Design review of the part built by this model. Coordinates are the model's own, in mm. Round coordinates to 2 decimals unless told otherwise and drop trailing zeros. Write each loop counter-clockwise with the first axis right and the second up, starting at its lowest first coordinate (ties: lowest second). Pieces come first, ordered by that corner, then holes. Notation, with made-up numbers: (22, -27) -> (39, -27) arc R19 ccw to (39, -2) -> close; hole circle Ø11 at (69.25, 80.25). An arc over 180 degrees is marked (long way). Write item = value, one per line. Start each with the question number.
Item 1: Add section B-B, the plane z = -600. State the section outline as (x, y) points, then the cut area to 3 significant figures.
Item 2: For pin 1 Ø1.9 at (y, z) = (3.5, -443.5) entering from -X; pin 2 Ø3 at (x, y) = (1036, 3.5) entering from -Z; pin 3 Ø11.5 at (x, z) = (22.225, -92.075) entering from -Y, all flat-tipped, find the tip position at first contact; note any pin that passes through.
Item 3: Add section C-C, the plane y = 3.5. State how many separate pieces and enclosed holes the cut face has, then the cut area to 3 significant figures.
Item 4: Add section D-D, the plane x = 881.5. State the section outline as (y, z) points (3 decimals).
Item 5: To check wall thickness, follow L1, parallel to X at y = 3.25, z = -309.5; L2, parallel to X at y = 0.75, z = -594.5; L3, parallel to X at y = 1, z = -278.5. State the ranges of each line that lie inside material, in increasing order.
Item 6: Add section A-A, the plane x = 88.9. State the section outline as (y, z) points (3 decimals).
from build123d import *

# Parameters (mm, degrees)
SKETCH1_R                                     = 3.3734375
BOSS_EXTRUDE1_DEPTH                           = 6.35
SKETCH3_R                                     = 2.45745
SKETCH3_R_2                                   = 22.225
CUT_EXTRUDE2_DEPTH                            = 1264.111411604
CUT_EXTRUDE1_DEPTH                            = 1264.111411604
CSK_FOR_1_4_FLAT_HEAD_MACHINE_SCREW1_AT_COUNT = 2
CSK_FOR_1_4_FLAT_HEAD_MACHINE_SCREW1_AT_PITCH = 1022.35
CSK_FOR_1_4_FLAT_HEAD_MACHINE_SCREW1_2_COUNT  = 2
CSK_FOR_1_4_FLAT_HEAD_MACHINE_SCREW1_2_PITCH  = 203.2
CSK_FOR_1_4_FLAT_HEAD_MACHINE_SCREW1_3_COUNT  = 2
CSK_FOR_1_4_FLAT_HEAD_MACHINE_SCREW1_3_PITCH  = 1042.348196382
FILLET1_R                                     = 6.35
FILLET3_R                                     = 3.175


with BuildPart() as part:
    # Sketch1 → Boss-Extrude1 (new body)
    with BuildSketch(Plane(origin=(0, 0, 0), x_dir=(1, 0, 0), z_dir=(0, 1, 0))):
        Polygon((1016, 406.4), (1066.8, 406.4), (1066.8, 0), (0, 0), (0, 406.4), (50.8, 406.4), (50.8, 530.225), (234.95, 530.225), (234.95, 676.275), (831.85, 676.275), (831.85, 530.225), (1016, 530.225), align=None)
        with Locations(Location((22.225, 92.075, 0), (0, 0, 270))):
            Circle(SKETCH1_R, mode=Mode.SUBTRACT)
        with Locations(Location((1044.575, 92.075, 0), (0, 0, 270))):
            Circle(SKETCH1_R, mode=Mode.SUBTRACT)
        with Locations(Location((22.225, 295.275, 0), (0, 0, 270))):
            Circle(SKETCH1_R, mode=Mode.SUBTRACT)
        with Locations(Location((1044.575, 295.275, 0), (0, 0, 270))):
            Circle(SKETCH1_R, mode=Mode.SUBTRACT)
    extrude(amount=BOSS_EXTRUDE1_DEPTH)

    # Sketch3 → Cut-Extrude2 (cut, through all)
    with BuildSketch(Plane(origin=(0, 6.35, 0), x_dir=(1, 0, 0), z_dir=(0, 1, 0))):
        with Locations(Location((134.9375, 487.748914195, 0), (0, 0, 270))):
            Circle(SKETCH3_R)
        with Locations(Location((219.486424299, 515.220524995, 0), (0, 0, 270))):
            Circle(SKETCH3_R)
        with Locations(Location((59.31154, 45.87748, 0), (0, 0, 270))):
            Circle(SKETCH3_R)
        with Locations(Location((296.845703608, 123.057008284, 0), (0, 0, 270))):
            Circle(SKETCH3_R)
        with Locations(Location((534.379867216, 200.236536569, 0), (0, 0, 270))):
            Circle(SKETCH3_R)
        with Locations(Location((771.914030824, 277.416064853, 0), (0, 0, 270))):
            Circle(SKETCH3_R)
        with Locations(Location((854.075, 309.0545, 0), (0, 0, 270))):
            Circle(SKETCH3_R)
        with Locations(Location((854.075, 486.8545, 0), (0, 0, 270))):
            Circle(SKETCH3_R)
        with Locations(Location((88.9, 492.125, 0), (0, 0, 270))):
            Circle(SKETCH3_R_2)
    extrude(amount=-CUT_EXTRUDE2_DEPTH, mode=Mode.SUBTRACT)

    # Sketch2 → Cut-Extrude1 (cut, through all)
    with BuildSketch(Plane(origin=(0, 6.35, 0), x_dir=(1, 0, 0), z_dir=(0, 1, 0))):
        Polygon((310.578822168, 0), (149.225, 0), (149.225, 95.25), (171.033618902, 121.240499926), (157.061866823, 164.241131286), (247.65, 193.675), align=None)
    extrude(amount=-CUT_EXTRUDE1_DEPTH, mode=Mode.SUBTRACT)

    # Sketch5 → CSK for 1/4 Flat Head Machine Screw1 (revolve, cut)
    with BuildSketch(Plane(origin=(22.225, 0, -92.075), x_dir=(0, 0, -1), z_dir=(1, 0, 0))):
        Polygon((0, 0), (0, 6.35), (3.3782, 6.35), (3.3782, 4.536932584), (6.4389, 1.016), (6.4389, 0), align=None)
    csk_for_1_4_flat_head_machine_screw1 = revolve(axis=Axis((22.225, -6.35, -92.075), (0, 1, 0)), mode=Mode.SUBTRACT)

    # CSK for 1/4 Flat Head Machine Screw1 at: CSK for 1/4 Flat Head Machine Screw1 ×2
    with Locations(*[(i * CSK_FOR_1_4_FLAT_HEAD_MACHINE_SCREW1_AT_PITCH, 0, 0) for i in range(1, CSK_FOR_1_4_FLAT_HEAD_MACHINE_SCREW1_AT_COUNT)]):
        add(csk_for_1_4_flat_head_machine_screw1, mode=Mode.SUBTRACT)

    # CSK for 1_4 Flat Head Machine Screw1 2: CSK for 1/4 Flat Head Machine Screw1 ×2
    with Locations(*[(0, 0, -i * CSK_FOR_1_4_FLAT_HEAD_MACHINE_SCREW1_2_PITCH) for i in range(1, CSK_FOR_1_4_FLAT_HEAD_MACHINE_SCREW1_2_COUNT)]):
        add(csk_for_1_4_flat_head_machine_screw1, mode=Mode.SUBTRACT)

    # CSK for 1_4 Flat Head Machine Screw1 3: CSK for 1/4 Flat Head Machine Screw1 ×2
    with Locations(*[Vector(0.9808142840837317, 0, -0.19494445397937524) * (i * CSK_FOR_1_4_FLAT_HEAD_MACHINE_SCREW1_3_PITCH) for i in range(1, CSK_FOR_1_4_FLAT_HEAD_MACHINE_SCREW1_3_COUNT)]):
        add(csk_for_1_4_flat_head_machine_screw1, mode=Mode.SUBTRACT)

    # Fillet1
    fillet1_edges = [part.edges().sort_by_distance(p)[0] for p in [
        (0, 3.175, -406.4),
        (50.8, 3.175, -406.4),
        (50.8, 3.175, -530.225),
        (234.95, 3.175, -530.225),
        (234.95, 3.175, -676.275),
        (831.85, 3.175, -676.275),
        (831.85, 3.175, -530.225),
        (1016, 3.175, -530.225),
        (1016, 3.175, -406.4),
        (1066.8, 3.175, -406.4),
        (1066.8, 3.175, 0),
        (0, 3.175, 0),
    ]]
    fillet(fillet1_edges, radius=FILLET1_R)

    # Fillet3
    fillet3_edges = [part.edges().sort_by_distance(p)[0] for p in [
        (247.65, 3.175, -193.675),
        (310.578822168, 3.175, 0),
        (149.225, 3.175, 0),
        (149.225, 3.175, -95.25),
        (171.033618902, 3.175, -121.240499926),
        (157.061866823, 3.175, -164.241131286),
    ]]
    fillet(fillet3_edges, radius=FILLET3_R)


solid = part.part
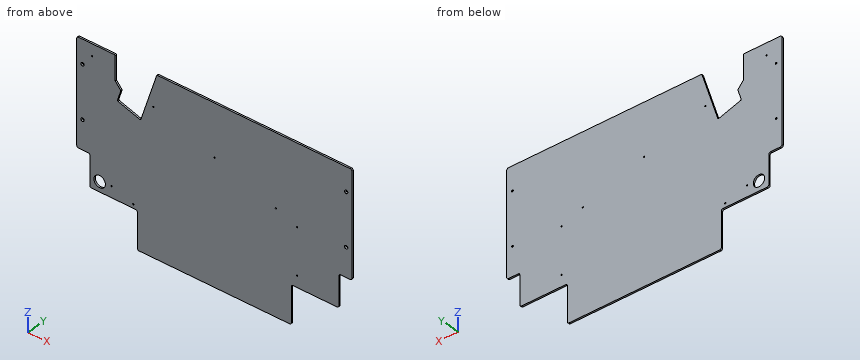
Result set:
q1.outline = (234.95, 0) -> (831.85, 0) -> (831.85, 6.35) -> (234.95, 6.35) -> close
q1.area = 3,790 mm²
q2.pin_1 = 50.8
q2.pin_2 = -406.4
q2.pin_3 = 1.81
q3.separate_pieces = 1
q3.enclosed_holes = 13
q3.area = 616,000 mm²
q4.outline = (0, -530.225) -> (6.35, -530.225) -> (6.35, 0) -> (0, 0) -> close
q5.L1 = 0 to 851.66, 856.49 to 1066.8
q5.L2 = 234.95 to 831.85
q5.L3 = 0 to 769.71, 774.12 to 1066.8
q6.outline = (0, -530.225) -> (6.35, -530.225) -> (6.35, -514.35) -> (0, -514.35) -> close; (0, -469.9) -> (6.35, -469.9) -> (6.35, 0) -> (0, 0) -> close
